Geometry: final body of the model. Coordinates: model frame, mm. Face numbers are marked on the shaded views. A direction names the side the tool comes from. Give positions to 0.01 mm unless a question says otherwise; leave off trailing zeros. Write each loop counter-clockwise with the first axis right and the second up, starting at its lowest first coordinate (ties: lowest second). Pieces come first, ordered by that corner, then holes.
Q1. Section D-D (z = 9). Return the cut outline in (x, y).
Q2. Reachability of the marked faces 1, 2, 3, 4 and 5 from +Z, -Z, +X, -X, +Y, -Y: full face, straight path, thin tool, end or side. Return the list, or none.
Q3. Section C-C (z = 30.5). Return the cut outline in (x, y).
Q4. Section A-A (x = 0). State how many separate pieces and enclosed holes the cut face has, plus the area to 3 significant figures.
Q5. Mould query, pull axis X, two halves, no side actions, for the marked faces 6, 7 and 8. Classes: +X half, -X half, draft (parallel to the pull), parting line (faces both ways), or undercut.
Q6. Section B-B (z = 17.5). Return the cut outline in (x, y).
Q7. Pin query (flat end, axial travel): pin 1 Ø13 at (x, y) = (4, -10) entering from +Z (3 decimals); pin 2 Ø1.3 at (y, z) = (37.5, 5) entering from -X; pin 3 Ø1.3 at (y, z) = (-36.5, 7.5) entering from -X; pin 4 Ø3 at (y, z) = (-41.5, 12.5) entering from +X. Return the tip coordinate at first contact, or that it passes through.
Q8. Line query: line 1 (Y direction, x = 0, z = 3.5); line 2 (X direction, y = 36.5, z = 11.25); line 3 (X direction, y = 36, z = 15). Output: solid intervals per line, ascending.
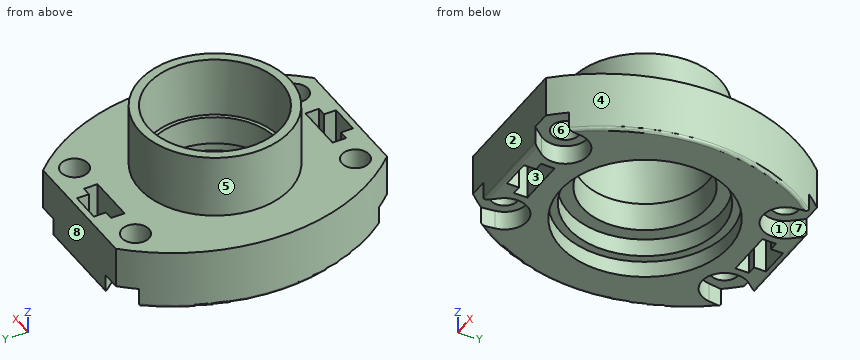
Autodesk Inventor part; units mm, degrees
ref_plane "EPANDOPPRO_XY" through (0, 0, 20) normal (0, 0, 1) x (1, 0, 0)
ref_plane "EPANDOPPRO_YZ" through (0, 0, 20) normal (1, 0, 0) x (0, 1, 0)
ref_plane "EPANDOPPRO_ZX" through (0, 0, 20) normal (0, 1, 0) x (0, 0, 1)
sketch "Skizze_1" plane through (0, 0, 0) normal (0, 0, 1) x (1, 0, 0)
  arc A0 (-21.5016, 45) -> (-21.5016, -45) centre (25.25, 0) ccw
  line L0 (-21.5016, -45) -> (21.5016, -45)
  arc A1 (21.5016, -45) -> (21.5016, 45) centre (-25.25, 0) ccw
  line L1 (21.5016, 45) -> (-21.5016, 45)
extrude "Extrusion1" add sketch "Skizze_1" along normal blind 20
sketch "Skizze_2" plane through (0, 0, 0) normal (0, 1, 0) x (-1, 0, 0)
  line L0 (-25.25, -50) -> (-25.25, 50)
  line L1 (40.14, -0.5) -> (40.14, 1)
  line L2 (40.14, 1) -> (39.64, 1)
  arc A0 (38.64, 0) -> (39.64, 1) centre (38.64, 1) ccw
  line L3 (38.64, 0) -> (38.64, -0.5)
  line L4 (38.64, -0.5) -> (40.14, -0.5)
revolve "Revolution1" cut sketch "Skizze_2" angle 360 about axis through (25.25, 0, -50) along (0, 0, -1)
sketch "Skizze_3" plane through (0, 0, 0) normal (0, 1, 0) x (-1, 0, 0)
  line L0 (25.25, 50) -> (25.25, -50)
  arc A0 (-39.64, 1) -> (-38.64, 0) centre (-38.64, 1) ccw
  line L1 (-39.64, 1) -> (-40.14, 1)
  line L2 (-40.14, 1) -> (-40.14, -0.5)
  line L3 (-40.14, -0.5) -> (-38.64, -0.5)
  line L4 (-38.64, -0.5) -> (-38.64, 0)
revolve "Revolution2" cut sketch "Skizze_3" angle 360 about axis through (-25.25, 0, 50) along (0, 0, 1)
sketch "Skizze_4" plane through (0, 0, 0) normal (1, 0, 0) x (0, 1, 0)
  arc A0 (44, 0) -> (45, 1) centre (44, 1) ccw
  line L0 (44, 0) -> (45, 0)
  line L1 (45, 0) -> (45, 1)
extrude "Extrusion2" cut sketch "Skizze_4" along normal mid plane 90
sketch "Skizze_5" plane through (0, 0, 0) normal (1, 0, 0) x (0, 1, 0)
  line L0 (-45, 1) -> (-45, 0)
  line L1 (-45, 0) -> (-44, 0)
  arc A0 (-45, 1) -> (-44, 0) centre (-44, 1) ccw
extrude "Extrusion3" cut sketch "Skizze_5" along normal mid plane 90
sketch "Skizze_6" plane through (0, 0, 0) normal (0, 0, 1) x (1, 0, 0)
  circle A0 centre (0, 0) radius 25
extrude "Extrusion4" add sketch "Skizze_6" along normal blind 41
sketch "Skizze_7" plane through (0, 0, 0) normal (0, 1, 0) x (-1, 0, 0)
  line L0 (0, 41) -> (0, 0)
  line L1 (0, 0) -> (-28, 0)
  line L2 (-28, 0) -> (-28, 5.5)
  line L3 (-28, 5.5) -> (-25.25, 5.5)
  line L4 (-25.25, 5.5) -> (-25.25, 11.5)
  line L5 (-25.25, 11.5) -> (-20.75, 11.5)
  line L6 (-20.75, 11.5) -> (-20.75, 21)
  line L7 (-20.75, 21) -> (-22, 21)
  line L8 (-22, 21) -> (-22, 41)
  line L9 (-22, 41) -> (0, 41)
  line L10 (0, 41) -> (0, 0)
revolve "Revolution3" cut sketch "Skizze_7" angle 360 about axis through (0, 0, 41) along (0, 0, 1)
sketch "Skizze_8" plane through (0, 0, 0) normal (0, 0, 1) x (1, 0, 0)
  line L0 (-8, 39) -> (-8, 34.5)
  line L1 (-8, 34.5) -> (8, 34.5)
  line L2 (8, 34.5) -> (8, 39)
  line L3 (8, 39) -> (5, 39)
  line L4 (5, 39) -> (5, 43)
  line L5 (5, 43) -> (-5, 43)
  line L6 (-5, 43) -> (-5, 39)
  line L7 (-5, 39) -> (-8, 39)
extrude "Extrusion5" cut sketch "Skizze_8" along normal blind 20
sketch "Skizze_9" plane through (0, 0, 0) normal (0, 0, 1) x (1, 0, 0)
  line L0 (-8, -34.5) -> (-8, -39)
  line L1 (-8, -39) -> (-5, -39)
  line L2 (-5, -39) -> (-5, -43)
  line L3 (-5, -43) -> (5, -43)
  line L4 (5, -43) -> (5, -39)
  line L5 (5, -39) -> (8, -39)
  line L6 (8, -39) -> (8, -34.5)
  line L7 (8, -34.5) -> (-8, -34.5)
extrude "Extrusion6" cut sketch "Skizze_9" along normal blind 20
sketch "Skizze_10" plane through (0, 0, 6.4) normal (0, 0, 1) x (1, 0, 0)
  circle A0 centre (18, 36.5) radius 4.5
extrude "Extrusion7" cut sketch "Skizze_10" along normal mid plane 40
pattern_linear "Rectangular Pattern1" count 2 spacing 36 along (-1, 0, 0) count 2 spacing 73 along (0, -1, 0) of "Extrusion7"
sketch "Skizze_12" plane through (0, 0, 6.4) normal (0, 0, 1) x (1, 0, 0)
  arc A0 (12.2226, 41.2825) -> (25.4357, 35.5199) centre (18, 36.5) ccw
  line L0 (25.4357, 35.5199) -> (26, 39.8014)
  arc A1 (26, 39.8014) -> (21.5016, 45) centre (-25.25, 0) ccw
  line L1 (21.5016, 45) -> (15.3, 45)
  line L2 (15.3, 45) -> (12.2226, 41.2825)
extrude "Extrusion8" cut sketch "Skizze_12" against normal blind 6.4
sketch "Skizze_13" plane through (0, 0, 6.4) normal (0, 0, 1) x (1, 0, 0)
  line L0 (-26, 39.8014) -> (-25.4357, 35.5199)
  arc A0 (-25.4357, 35.5199) -> (-12.2226, 41.2825) centre (-18, 36.5) ccw
  line L1 (-12.2226, 41.2825) -> (-15.3, 45)
  line L2 (-15.3, 45) -> (-21.5016, 45)
  arc A1 (-21.5016, 45) -> (-26, 39.8014) centre (25.25, 0) ccw
extrude "Extrusion9" cut sketch "Skizze_13" against normal blind 6.4
sketch "Skizze_14" plane through (0, 0, 6.4) normal (0, 0, 1) x (1, 0, 0)
  arc A0 (25.4357, -35.5199) -> (12.2226, -41.2825) centre (18, -36.5) ccw
  line L0 (12.2226, -41.2825) -> (15.3, -45)
  line L1 (15.3, -45) -> (21.5016, -45)
  arc A1 (21.5016, -45) -> (26, -39.8014) centre (-25.25, 0) ccw
  line L2 (26, -39.8014) -> (25.4357, -35.5199)
extrude "Extrusion10" cut sketch "Skizze_14" against normal blind 6.4
sketch "Skizze_15" plane through (0, 0, 6.4) normal (0, 0, 1) x (1, 0, 0)
  arc A0 (-26, -39.8014) -> (-21.5016, -45) centre (25.25, 0) ccw
  line L0 (-21.5016, -45) -> (-15.3, -45)
  line L1 (-15.3, -45) -> (-12.2226, -41.2825)
  arc A1 (-12.2226, -41.2825) -> (-25.4357, -35.5199) centre (-18, -36.5) ccw
  line L2 (-25.4357, -35.5199) -> (-26, -39.8014)
extrude "Extrusion11" cut sketch "Skizze_15" against normal blind 6.4
ref_plane "EPANDOPPRO_XY" through (0, 0, 20) normal (0, 0, 1) x (1, 0, 0)
ref_plane "EPANDOPPRO_YZ" through (0, 0, 20) normal (1, 0, 0) x (0, 1, 0)
ref_plane "EPANDOPPRO_ZX" through (0, 0, 20) normal (0, 1, 0) x (0, 0, 1)
ref_plane "EPDICHTR_XY" through (0, 0, 5.5) normal (0, 0, 1) x (1, 0, 0)
ref_plane "EPDICHTR_YZ" through (0, 0, 5.5) normal (1, 0, 0) x (0, 1, 0)
ref_plane "EPDICHTR_ZX" through (0, 0, 5.5) normal (0, 1, 0) x (0, 0, 1)
ref_plane "EPZYL_XY" through (18, 36.5, 6.4) normal (0, 0, 1) x (1, 0, 0)
ref_plane "EPZYL_YZ" through (18, 36.5, 6.4) normal (1, 0, 0) x (0, 1, 0)
ref_plane "EPZYL_ZX" through (18, 36.5, 6.4) normal (0, 1, 0) x (0, 0, 1)
ref_plane "EPZYL2_XY" through (-18, 36.5, 6.4) normal (0, 0, 1) x (1, 0, 0)
ref_plane "EPZYL2_YZ" through (-18, 36.5, 6.4) normal (1, 0, 0) x (0, 1, 0)
ref_plane "EPZYL2_ZX" through (-18, 36.5, 6.4) normal (0, 1, 0) x (0, 0, 1)
ref_plane "EPZYL3_XY" through (-18, -36.5, 6.4) normal (0, 0, 1) x (1, 0, 0)
ref_plane "EPZYL3_YZ" through (-18, -36.5, 6.4) normal (1, 0, 0) x (0, 1, 0)
ref_plane "EPZYL3_ZX" through (-18, -36.5, 6.4) normal (0, 1, 0) x (0, 0, 1)
ref_plane "EPZYL4_XY" through (18, -36.5, 6.4) normal (0, 0, 1) x (1, 0, 0)
ref_plane "EPZYL4_YZ" through (18, -36.5, 6.4) normal (1, 0, 0) x (0, 1, 0)
ref_plane "EPZYL4_ZX" through (18, -36.5, 6.4) normal (0, 1, 0) x (0, 0, 1)
properties part number "Abdeckkappe_LZ80"
Computed:
1. outline: (-21.5, -45) - (21.5, -45) arc R64.89 ccw to (21.5, 45) - (-21.5, 45) arc R64.89 ccw to start; hole circle Ø50.5 at (0, 0); hole circle Ø9 at (-18, -36.5); hole circle Ø9 at (-18, 36.5); hole (-8, -39) - (-5, -39) - (-5, -43) - (5, -43) - (5, -39) - (8, -39) - (8, -34.5) - (-8, -34.5) - close; hole (-8, 34.5) - (8, 34.5) - (8, 39) - (5, 39) - (5, 43) - (-5, 43) - (-5, 39) - (-8, 39) - close; hole circle Ø9 at (18, -36.5); hole circle Ø9 at (18, 36.5)
2. face 1: -Z
2. face 2: +Z, -Z, +X, -X, -Y
2. face 3: +Z, -Z
2. face 4: +Z, -Z, +X
2. face 5: +Z
3. outline: circle Ø50 at (0, 0); hole circle Ø44 at (0, 0)
4. separate pieces: 4
4. enclosed holes: 0
4. area: 624 mm2
5. face 6: undercut
5. face 7: +X half
5. face 8: draft
6. outline: (-21.5, -45) - (21.5, -45) arc R64.89 ccw to (21.5, 45) - (-21.5, 45) arc R64.89 ccw to start; hole circle Ø9 at (-18, -36.5); hole circle Ø9 at (-18, 36.5); hole circle Ø41.5 at (0, 0); hole (-8, -39) - (-5, -39) - (-5, -43) - (5, -43) - (5, -39) - (8, -39) - (8, -34.5) - (-8, -34.5) - close; hole (-8, 34.5) - (8, 34.5) - (8, 39) - (5, 39) - (5, 43) - (-5, 43) - (-5, 39) - (-8, 39) - close; hole circle Ø9 at (18, -36.5); hole circle Ø9 at (18, 36.5)
7. pin 1: passes through
7. pin 2: stops at x = -28.16
7. pin 3: stops at x = -28.84
7. pin 4: stops at x = 25.85
8. line 1: y = -45 to -43, -34.5 to -28, 28 to 34.5, 43 to 45
8. line 2: x = -28.4 to -22.5, -13.5 to -8, 8 to 13.5, 22.5 to 28.4
8. line 3: x = -28.74 to -22.47, -13.53 to -8, 8 to 13.53, 22.47 to 28.74
